Autodesk Fusion 360 part; units mm, degrees
sketch "Sketch1" plane through (0, 0, 0) normal (0, 0, 1) x (1, 0, 0)
  line L0 (0, 0) -> (2, 0)
  line L1 (2, 0) -> (6, 0)
  line L2 (6, 0) -> (6, 10)
  line L3 (6, 10) -> (10, 10)
  line L4 (10, 10) -> (10, 0)
  line L5 (10, 0) -> (24, 0)
  line L6 (24, 0) -> (24, 10)
  line L7 (24, 10) -> (28, 10)
  line L8 (28, 10) -> (28, 0)
  line L9 (28, 0) -> (32, 0)
  line L10 (32, 0) -> (34, 0)
  line L11 (34, 0) -> (34, 2)
  line L12 (34, 2) -> (32, 2)
  line L13 (32, 2) -> (32, 27)
  line L14 (0, 0) -> (0, 2)
  line L15 (0, 2) -> (2, 2)
  line L16 (2, 2) -> (2, 27)
  line L17 (2, 27) -> (32, 27)
  line L18 (2, 2) -> (2, 0)
  line L19 (32, 2) -> (32, 0)
  dimension "d1" = 2
  dimension "d2" = 4
  dimension "d3" = 10
  dimension "d4" = 4
  dimension "d5" = 14
  dimension "d6" = 4
  dimension "d7" = 4
  dimension "d8" = 2
  dimension "d9" = 2
  dimension "d10" = 2
  dimension "d11" = 25
  dimension "d12" = 2
  dimension "d13" = 2
  dimension "d14" = 25
  dimension "d43" = 30
extrude "Extrude1" add sketch "Sketch1" along normal blind 4 contours L1 L2 L3 L4 L5 L6 L7 L8 L9 L13 L16 L17 L18 L19
sketch "Sketch2" plane through (32, 0, 0) normal (1, 0, 0) x (0, 1, 0)
  line L0 (0, 0) -> (27, 0)
  line L1 (27, 0) -> (27, 4)
  line L2 (27, 4) -> (0, 4)
  line L3 (0, 4) -> (0, 0)
  circle A0 centre (4, 2) radius 1
  dimension "d17" = 2
  dimension "d56" = 2
  dimension "d57" = 4
sketch "Sketch3" plane through (32, 0, 0) normal (1, 0, 0) x (0, 1, 0)
  line L0 (0, 4) -> (0, 0)
  line L1 (0, 4) -> (0, 2)
  line L2 (0, 2) -> (4.8814, 2)
  point P0 (0, 4)
extrude "Extrude2" add sketch "Sketch2" along normal blind 3 contours A0
sketch "Sketch4" plane through (2, 0, 0) normal (-1, 0, 0) x (0, -1, 0)
  line L0 (-27, 0) -> (0, 0)
  line L1 (0, 0) -> (0, 4)
  line L2 (0, 4) -> (-27, 4)
  line L3 (-27, 4) -> (-27, 0)
  circle A0 centre (-4, 2) radius 1
  line L4 (0, 0) -> (0, 2)
  dimension "d20" = 2
  dimension "d54" = 2
  dimension "d55" = 4
extrude "Extrude3" add sketch "Sketch4" along normal blind 3 contours A0
fillet "Fillet1" radius 2.5 1 edges at (17, 27, 4)
sketch "Sketch5" plane through (0, 0, 4) normal (0, 0, 1) x (-1, 0, 0)
  line L0 (-32, -24.5) -> (-2, -24.5)
  line L1 (-2, -24.5) -> (-2, 0)
  line L2 (-2, 0) -> (-6, 0)
  line L3 (-6, 0) -> (-6, -10)
  line L4 (-6, -10) -> (-10, -10)
  line L5 (-10, -10) -> (-10, 0)
  line L6 (-10, 0) -> (-24, 0)
  line L7 (-24, 0) -> (-24, -10)
  line L8 (-24, -10) -> (-28, -10)
  line L9 (-28, -10) -> (-28, 0)
  line L10 (-28, 0) -> (-32, 0)
  line L11 (-32, 0) -> (-32, -24.5)
  line L12 (-28, -6.2874) -> (-16.9, -6.2874)
  line L13 (-16.9, -6.2874) -> (-16.9, -24.5)
  line L14 (-16.9, -24.5) -> (-28, -24.5)
  line L15 (-28, -24.5) -> (-28, -6.2874)
extrude "Extrude4" cut sketch "Sketch5" against normal blind 2 contours L0 L7 L8 L12 L13 L14 L15
fillet "Fillet2" radius 1.5 1 edges at (17, 0, 4)
fillet "Fillet3" radius 1.5 1 edges at (4, 0, 4)
fillet "Fillet4" radius 1.5 1 edges at (30, 0, 4)
sketch "Sketch6" plane through (0, 0, 2) normal (0, 0, 1) x (-1, 0, 0)
  line L0 (-16.9, -6.2874) -> (-24, -6.2874)
  line L1 (-24, -6.2874) -> (-24, -10)
  line L2 (-24, -10) -> (-28, -10)
  line L3 (-28, -10) -> (-28, -24.5)
  line L4 (-28, -24.5) -> (-16.9, -24.5)
  line L5 (-16.9, -24.5) -> (-16.9, -6.2874)
  line L6 (-28, -24.5) -> (-3.7012, -24.5)
  line L7 (-3.7012, -24.5) -> (-3.7012, -19.6935)
  line L8 (-28, -19.6935) -> (-28, -24.5)
extrude "Extrude6" add sketch "Sketch6" along normal blind 2
fillet "Fillet9" radius 1.5 2 edges at (10, 10, 2) (24, 10, 2)
extrude "Extrude5" add sketch "Sketch6" along normal blind 2
sketch "Sketch7" plane through (0, 0, 4) normal (0, 0, 1) x (-1, 0, 0)
  line L0 (-28, -10) -> (-28, -1.5)
  line L1 (-28, -1.5) -> (-32, -1.5)
  line L2 (-32, -1.5) -> (-32, -24.5)
  line L3 (-32, -24.5) -> (-2, -24.5)
  line L4 (-2, -24.5) -> (-2, -1.5)
  line L5 (-2, -1.5) -> (-6, -1.5)
  line L6 (-6, -1.5) -> (-6, -10)
  line L7 (-6, -10) -> (-8.5, -10)
  arc A0 (-10, -8.5) -> (-8.5, -10) centre (-8.5, -8.5) ccw
  line L8 (-10, -8.5) -> (-10, -1.5)
  line L9 (-10, -1.5) -> (-24, -1.5)
  line L10 (-24, -1.5) -> (-24, -8.5)
  arc A1 (-25.5, -10) -> (-24, -8.5) centre (-25.5, -8.5) ccw
  line L11 (-25.5, -10) -> (-28, -10)
  line L12 (-24, -4) -> (-10, -4)
  line L13 (-28, -10) -> (-28, -22)
  line L14 (-28, -22) -> (-6, -22)
  line L15 (-6, -22) -> (-6, -10)
extrude "Extrude7" cut sketch "Sketch7" against normal blind 2 contours L7 A0 L8 L10 A1 L11 L12 L13 L14 L15
extrude "Extrude8" add 1 faces at (20.6667, 22, 3.3333) along direction (0, -1, 0) blind 1
fillet "Fillet10" radius 1.5 2 edges at (6, 21, 3) (28, 21, 3)
fillet "Fillet11" radius 2.5 3 edges at (17, 0, 0) (4, 0, 0) (30, 0, 0)
fillet "Fillet12" radius 1.25 1 edges at (17, 4, 4)
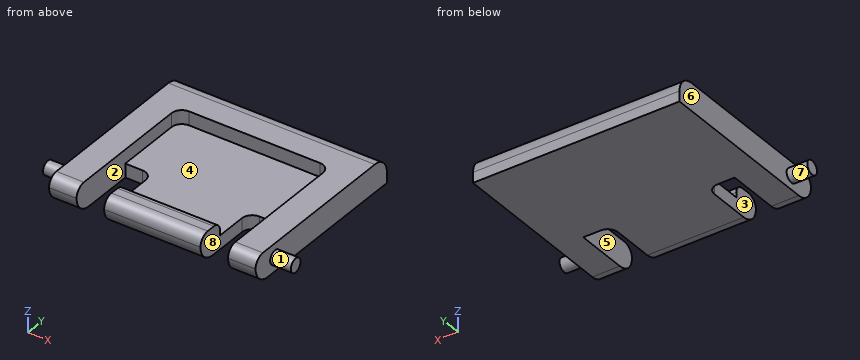
Part model, mm, in its own coordinate system. Face numbers are marked on the shaded views. A direction names the side the tool comes from. Coordinates: 2 decimals unless noted, no trailing zeros. Order: outer loops, then holes, each group sorted by start corner. A loop starts at its lowest first (then second) coordinate and runs counter-clockwise, first axis right, second up. Notation, with made-up numbers: M 82.5,-4.75 L 112.5,-4.75 A21 ccw 112.5,11.25 Z; hole C -23,-27 d11. An arc over 180 degrees is marked long. Use a Markdown table: item, result.
(1) Cut at C-C on y = 13.75. Write the cut outline in (x, z).
A:
| item | result |
|---|---|
| outline | M 2,0 L 32,0 L 32,4 L 28,4 L 28,2 L 6,2 L 6,4 L 2,4 Z |
(2) Pull direction X, two halves, no side cores. Call the marked faces 5, 6, 7 and 8: released by +X, released by -X, zero draft, split by the parting line, or undercut.
A:
| item | result |
|---|---|
| face 5 | undercut |
| face 6 | released by -X |
| face 7 | zero draft |
| face 8 | undercut |
(3) Probe L1, parallel to X at y = 3, z = 3.4; L2, parallel to X at y = 16.25, z = 3.65; L3, parallel to Z at x = 15, y = 16.5. List the from-to ranges inside material, lowest first.
A:
| item | result |
|---|---|
| L1 | x = 2 to 6, 10 to 24, 28 to 32 |
| L2 | x = 2 to 6, 28 to 32 |
| L3 | z = 0 to 2 |
(4) Tool access for the marked faces 1, 2, 3 and 4: list every direction of +Z, -Z, +X, -X, +Y, -Y with a clear straight run to the whole face (end or side of a thin tool).
A:
| item | result |
|---|---|
| face 1 | +X |
| face 2 | +Z, -Y |
| face 3 | +Z, -Z, -Y |
| face 4 | +Z |
(5) Cut at A-A on z = 3.45. Write the cut outline in (x, y), then the cut area to 3 significant figures.
A:
| item | result |
|---|---|
| outline | M 2,0.34 L 6,0.34 L 6,19.5 A1.5 cw 7.5,21 L 26.5,21 A1.5 cw 28,19.5 L 28,0.34 L 32,0.34 L 32,26.06 L 2,26.06 Z; M 10,0.34 L 24,0.34 L 24,3.79 L 10,3.79 Z |
| area | 366 mm^2 |
(6) Flat gauge pins, fed straight in: pin 1 (8 mm diameter, centred on x = 14, y = 15, fed in from +Z); pin 2 (1 mm diameter, centred on y = 7, z = 1, fed in from -X); pin 3 (0.6 mm diameter, centred on x = 19, z = 3, fed in from -Y). Where does each tip first touch, or does it go through?
A:
| item | result |
|---|---|
| pin 1 | stops at z = 2 |
| pin 2 | stops at x = 2 |
| pin 3 | stops at y = 0.01 |
